```python
from build123d import *

# Parameters (mm, degrees)
BOSS_EXTRUDE1_DEPTH   = 50
BOSS_EXTRUDE2_DEPTH   = 50
BOSS_EXTRUDE2_2_DEPTH = 50
SKETCH3_W             = 100
SKETCH3_H             = 20
BOSS_EXTRUDE2_3_DEPTH = 50
SKETCH4_W             = 60
SKETCH4_H             = 20
CUT_EXTRUDE1_DEPTH    = 50
FILLET1_R             = 10
FILLET2_R             = 10
FILLET3_R             = 10
FILLET4_R             = 10
FILLET5_R             = 10
FILLET6_R             = 10
FILLET7_R             = 10
SKETCH5_R             = 5
BOSS_EXTRUDE3_DEPTH   = 80
SKETCH6_R             = 5
BOSS_EXTRUDE4_DEPTH   = 80


with BuildPart() as part:
    # Sketch1 → Boss-Extrude1 (new body)
    with BuildSketch(Plane(origin=(0, 0, 0), x_dir=(1, 0, 0), z_dir=(0, 1, 0))):
        Polygon((-190.55, -110), (190.55, -110), (0, 220.042281382), align=None)
    extrude(amount=BOSS_EXTRUDE1_DEPTH)


with BuildPart() as body_2:
    # Sketch3 → Boss-Extrude2 (new body)
    with BuildSketch(Plane(origin=(0, 0, 0), x_dir=(1, 0, 0), z_dir=(0, 1, 0))):
        Polygon((-128.935254038, 16.719870502), (-111.614745962, 6.719870502), (-61.614745962, 93.32241088), (-78.935254038, 103.32241088), align=None)
    extrude(amount=BOSS_EXTRUDE2_DEPTH)


with BuildPart() as body_3:
    # Sketch3 → Boss-Extrude2 2 (new body)
    with BuildSketch(Plane(origin=(0, 0, 0), x_dir=(1, 0, 0), z_dir=(0, 1, 0))):
        Polygon((111.614745962, 6.719870502), (61.614745962, 93.32241088), (78.935254038, 103.32241088), (128.935254038, 16.719870502), align=None)
    extrude(amount=BOSS_EXTRUDE2_2_DEPTH)


with BuildPart() as body_4:
    # Sketch3 → Boss-Extrude2 3 (new body)
    with BuildSketch(Plane(origin=(0, 0, 0), x_dir=(1, 0, 0), z_dir=(0, 1, 0))):
        with Locations((0, -110)):
            Rectangle(SKETCH3_W, SKETCH3_H)
    extrude(amount=BOSS_EXTRUDE2_3_DEPTH)


with BuildPart() as body_2_1:
    # Body-Move/Copy1: read off the stored shape, not the designer's step
    # Body-Move/Copy1: moved
    add(body_2.part.moved(Location((-8.660254, 0, -5))))


with BuildPart() as body_3_1:
    # Body-Move/Copy2: read off the stored shape, not the designer's step
    # Body-Move/Copy2: moved
    add(body_3.part.moved(Location((8.660254, 0, -5))))


with BuildPart() as body_4_1:
    # Body-Move/Copy3: read off the stored shape, not the designer's step
    # Body-Move/Copy3: moved
    add(body_4.part.moved(Location((0, 0, 10))))


with BuildPart() as cut_extrude1_tool:
    # Sketch4 → Cut-Extrude1 (new body)
    with BuildSketch(Plane(origin=(0, 50, 0), x_dir=(1, 0, 0), z_dir=(0, 1, 0))):
        Polygon((-97.595508076, 91.001902805), (-80.275, 81.001902805), (-110.275, 29.040378578), (-127.595508076, 39.040378578), align=None)
        Polygon((127.595508076, 39.040378578), (97.595508076, 91.001902805), (80.275, 81.001902805), (110.275, 29.040378578), align=None)
        with Locations((0, -120)):
            Rectangle(SKETCH4_W, SKETCH4_H)
    extrude(amount=-CUT_EXTRUDE1_DEPTH)


with BuildPart() as body_2_2:
    add(body_2_1.part)

    # Cut-Extrude1: cut by cut_extrude1_tool
    add(cut_extrude1_tool.part, mode=Mode.SUBTRACT)


with BuildPart() as body_3_2:
    add(body_3_1.part)

    # Cut-Extrude1: cut by cut_extrude1_tool
    add(cut_extrude1_tool.part, mode=Mode.SUBTRACT)


with BuildPart() as body_4_2:
    add(body_4_1.part)

    # Cut-Extrude1: cut by cut_extrude1_tool
    add(cut_extrude1_tool.part, mode=Mode.SUBTRACT)


with BuildPart() as cut_extrude1_piece_1:
    # of the separate pieces the step leaves, piece 1, a body of its own (cut_extrude1_pieces)
    add(body_2_2.part.solids().sort_by_distance((-87.595508038, 0, -108.32241088))[0])

    # Fillet1
    fillet1_edges = [cut_extrude1_piece_1.edges().sort_by_distance(p)[0] for p in [
        (-92.595508043, 0, -99.662156834),
        (-92.595508043, 50, -99.662156834),
    ]]
    fillet(fillet1_edges, radius=FILLET1_R)


with BuildPart() as cut_extrude1_piece_2:
    # of the separate pieces the step leaves, piece 2, a body of its own (cut_extrude1_pieces)
    add(body_2_2.part.solids().sort_by_distance((-137.595508038, 0, -21.719870502))[0])

    # Fillet2
    fillet2_edges = [cut_extrude1_piece_2.edges().sort_by_distance(p)[0] for p in [
        (-132.595508043, 0, -30.380124532),
        (-132.595508043, 50, -30.380124532),
    ]]
    fillet(fillet2_edges, radius=FILLET2_R)


with BuildPart() as cut_extrude1_piece_1_of_body_3:
    # of the separate pieces the step leaves, piece 1, a body of its own (cut_extrude1_pieces_of_body_3)
    add(body_3_2.part.solids().sort_by_distance((80.275, 0, -81.001902805))[0])

    # Fillet7
    fillet7_edges = [cut_extrude1_piece_1_of_body_3.edges().sort_by_distance(p)[0] for p in [
        (92.595508043, 0, -99.662156834),
        (92.595508043, 50, -99.662156834),
    ]]
    fillet(fillet7_edges, radius=FILLET7_R)


with BuildPart() as cut_extrude1_piece_2_of_body_3:
    # of the separate pieces the step leaves, piece 2, a body of its own (cut_extrude1_pieces_of_body_3)
    add(body_3_2.part.solids().sort_by_distance((120.274999962, 0, -11.719870502))[0])

    # Fillet6
    fillet6_edges = [cut_extrude1_piece_2_of_body_3.edges().sort_by_distance(p)[0] for p in [
        (132.595508043, 0, -30.380124532),
        (132.595508043, 50, -30.380124532),
    ]]
    fillet(fillet6_edges, radius=FILLET6_R)


with BuildPart() as cut_extrude1_piece_1_of_body_4:
    # of the separate pieces the step leaves, piece 1, a body of its own (cut_extrude1_pieces_of_body_4)
    add(body_4_2.part.solids().sort_by_distance((50, 0, 110))[0])

    # Fillet5
    fillet5_edges = [cut_extrude1_piece_1_of_body_4.edges().sort_by_distance(p)[0] for p in [
        (40, 0, 130),
        (40, 50, 130),
    ]]
    fillet(fillet5_edges, radius=FILLET5_R)


with BuildPart() as cut_extrude1_piece_2_of_body_4:
    # of the separate pieces the step leaves, piece 2, a body of its own (cut_extrude1_pieces_of_body_4)
    add(body_4_2.part.solids().sort_by_distance((-30, 0, 110))[0])

    # Fillet3
    fillet3_edges = [cut_extrude1_piece_2_of_body_4.edges().sort_by_distance(p)[0] for p in [
        (-40, 50, 130),
    ]]
    fillet(fillet3_edges, radius=FILLET3_R)

    # Fillet4
    fillet4_edges = [cut_extrude1_piece_2_of_body_4.edges().sort_by_distance(p)[0] for p in [
        (-40, 0, 130),
    ]]
    fillet(fillet4_edges, radius=FILLET4_R)


with BuildPart() as cut_extrude1_piece_2_of_body_3_1:
    add(cut_extrude1_piece_2_of_body_3.part)

    # Combine1: union Cut-Extrude1 piece 2, Cut-Extrude1 piece 2 of body 4, part, Cut-Extrude1 piece 1 of body 4, Cut-Extrude1 piece 1, Cut-Extrude1 piece 1 of body 3
    add(cut_extrude1_piece_2.part)
    add(cut_extrude1_piece_2_of_body_4.part)
    add(part.part)
    add(cut_extrude1_piece_1_of_body_4.part)
    add(cut_extrude1_piece_1.part)
    add(cut_extrude1_piece_1_of_body_3.part)


with BuildPart() as body_2_2_1:
    # Sketch5 → Boss-Extrude3 (new body)
    with BuildSketch(Plane(origin=(-24.993897208, 0, 43.290699844), x_dir=(0.8660254037844362, 0, 0.5000000000000046), z_dir=(-0.5000000000000044, 0, 0.866025403784436))):
        with Locations((-120.021140691, 25)):
            Circle(SKETCH5_R)
    extrude(amount=-BOSS_EXTRUDE3_DEPTH)


with BuildPart() as body_3_2_1:
    # Mirror3: mirrored copy
    add(body_2_2_1.part.mirror(Plane(origin=(0, 0, 0), x_dir=(0, 0, 1), z_dir=(1, 0, 0))))


with BuildPart() as body_2_2_2:
    add(body_2_2_1.part)

    # Combine2: union body 3 2, Cut-Extrude1 piece 2 of body 3
    add(body_3_2_1.part)
    add(cut_extrude1_piece_2_of_body_3_1.part)

    # Sketch6 → Boss-Extrude4 (add)
    with BuildSketch(Plane.ZY.offset(50)):
        with Locations((120, 25)):
            Circle(SKETCH6_R)
    extrude(amount=-BOSS_EXTRUDE4_DEPTH)


solid = body_2_2_2.part
```
The listing builds one solid part. Answer for the finished solid, in the listing's coordinates (mm). A direction names the side the tool comes from. Give positions to 0.01 mm unless a question says otherwise; leave off trailing zeros. Order: outer loops, then holes, each group sorted by start corner. A loop starts at its lowest first (then second) coordinate and runs counter-clockwise, first axis right, second up.
Item 1: The part is cut by section B-B, the plane z = 8. Give the vertices of the cut face in (x, y), and give its area (3 significant figures).
From the geometry:
outline: (-131.66, 0) - (131.66, 0) - (131.66, 50) - (-131.66, 50) - close
area: 13,200 mm2
Item 2: The part is cut by section A-A, the plane x = 17.5. Give the vertices of the cut face in (y, z).
From the geometry:
outline: (0, -189.73) - (50, -189.73) - (50, 110) - (0, 110) - close; circle Ø10 at (25, 120)
Item 3: The part is cut by section D-D, the plane y = 25. Count the separate pieces of the cut face and the enclosed holes in it, and give its area (3 significant figures).
From the geometry:
separate pieces: 1
enclosed holes: 3
area: 67,100 mm2
Item 4: Given pin 1 Ø6 at (x, y) = (-17.5, 39.5) entering from -Z; pin 2 Ø15 at (x, y) = (-133, 23) entering from +Z; pin 3 Ø10 at (x, y) = (-28.5, 5.5) entering from -Z, each flat-ended and moving along its own axis, determine where each tip first touches the part or whether it passes through.
From the geometry:
pin 1: stops at z = -194.93
pin 2: stops at z = 110
pin 3: stops at z = -179.34
Item 5: The part is cut by section C-C, the plane x = -157. Give the vertices of the cut face in (y, z), and give its area (3 significant figures).
From the geometry:
outline: (0, 51.89) - (50, 51.89) - (50, 110) - (0, 110) - close
area: 2,910 mm2
Item 6: Which of the six approach directions +Z, -Z, +X, -X, +Y, -Y give full straight-line access (tool end or side, diameter ignored) to faces 1 (the face through (-78.81, 24.65, -103.25)), 2 (the face through (95.485, 24.65, -54.657)), 3 (the face through (-121, 25, 110)), 4 (the face through (-0.42, 20.564, 122.307))?
From the geometry:
face 1: -Z, +Y, -Y
face 2: +Y, -Y
face 3: +Z, -X, +Y, -Y
face 4: none
Item 7: Find the intervals of material crossed by probe 1 along Z at (x, y) = (95.5, 25); probe 2 along X at (y, z) = (14, -13.5); probe 3 along X at (y, z) = (27, -39.5), in increasing order.
From the geometry:
probe 1: z = -94.63 to -89.79, -84.63 to -64.63, -54.63 to 110
probe 2: x = -123.36 to 123.36
probe 3: x = -121.07 to -110.49, -104.24 to 104.24, 110.49 to 121.07
Item 8: For a pull along X with two mould halves and no side action, classify faces 5 (the face through (-130.2, 46.99, -28.83)), 6 (the face through (-118.81, 30.91, -33.97)), 7 (the face through (40, 25, 130)) as pulls with the +X half, pulls with the -X half, needs draft (parallel to the pull), parting line crosses it, or undercut.
From the geometry:
face 5: pulls with the -X half
face 6: undercut
face 7: needs draft
